For this review, take the finished solid that the model builds, in its own axes (mm). Face numbers are marked on the shaded views. A direction names the side the tool comes from. Round coordinates to 2 decimals unless told otherwise and drop trailing zeros. Order: outer loops, then holes, each group sorted by start corner. A loop starts at its lowest first (then second) coordinate and runs counter-clockwise, first axis right, second up.
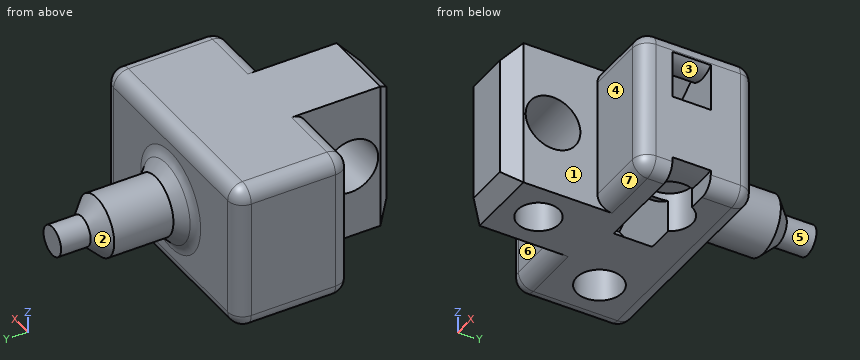
```python
from build123d import *

# Parameters (mm, degrees)
ESBO_O2_W                     = 100
ESBO_O2_H                     = 60
RESSALTO_EXTRUS_O1_DEPTH      = 50
RESSALTO_EXTRUS_O2_DEPTH      = 50
RESSALTO_EXTRUS_O2_DEPTH_BACK = 100
ESBO_O3_W                     = 100
ESBO_O3_H                     = 76.966331483
ESBO_O4_R                     = 20
RESSALTO_EXTRUS_O3_DEPTH      = 60
FILETE1_R                     = 10
CHANFRO1_SIZE                 = 10
ESBO_O6_R                     = 18.5
CORTE_EXTRUS_O1_DEPTH         = 243.47832014
ESBO_O7_R                     = 14.082818634
ESBO_O7_R_2                   = 15.375713497
CORTE_EXTRUS_O2_DEPTH         = 27
ESBO_O8_R                     = 10
RESSALTO_EXTRUS_O4_DEPTH      = 20
FILETE2_R                     = 10
CHANFRO2_SIZE                 = 10
ESBO_O10_W                    = 27.587633248
ESBO_O10_H                    = 25.966331483
ESBO_O10_W_2                  = 29.412366752
CORTE_REVOLU_O1_ANGLE         = 325


with BuildPart() as part:
    # Esboço2 → Ressalto-extrusão1 (new body)
    with BuildSketch(Plane(origin=(0, 0, 0), x_dir=(0, 0, -1), z_dir=(1, 0, 0))):
        with Locations((50, 30)):
            Rectangle(ESBO_O2_W, ESBO_O2_H)
    extrude(amount=RESSALTO_EXTRUS_O1_DEPTH)

    # Esboço3 → Ressalto-extrusão2 (add, two sides: drawn at the far end of the back side and taken through both)
    with BuildSketch(Plane.ZY.offset(-RESSALTO_EXTRUS_O2_DEPTH_BACK)):
        with Locations((-50, 98.483165742)):
            Rectangle(ESBO_O3_W, ESBO_O3_H)
    extrude(amount=RESSALTO_EXTRUS_O2_DEPTH + RESSALTO_EXTRUS_O2_DEPTH_BACK)

    # Esboço4 → Ressalto-extrusão3 (add)
    with BuildSketch(Plane(origin=(0, 136.966331483, 0), x_dir=(1, 0, 0), z_dir=(0, 1, 0))):
        with Locations(Location((25, 50, 0), (0, 0, 90))):
            Circle(ESBO_O4_R)
    extrude(amount=RESSALTO_EXTRUS_O3_DEPTH)

    # Filete1
    filete1_edges = [part.edges().sort_by_distance(p)[0] for p in [
        (-25, 60, -100),
        (75, 60, -100),
        (100, 60, -50),
        (-25, 60, 0),
        (75, 60, 0),
        (100, 98.483165742, 0),
        (25, 136.966331483, 0),
        (100, 136.966331483, -50),
        (25, 136.966331483, -100),
        (100, 98.483165742, -100),
        (-50, 60, -50),
        (-50, 98.483165742, 0),
        (-50, 136.966331483, -50),
        (-50, 98.483165742, -100),
    ]]
    fillet(filete1_edges, radius=FILETE1_R)

    # Chanfro1
    chanfro1_edges = [part.edges().sort_by_distance(p)[0] for p in [
        (25, 136.966331483, -30),
        (25, 196.966331483, -30),
    ]]
    chamfer(chanfro1_edges, length=CHANFRO1_SIZE)

    # Esboço6 → Corte-extrusão1 (cut, through all)
    with BuildSketch(Plane(origin=(50, 0, 0), x_dir=(0, 0, -1), z_dir=(1, 0, 0))):
        with Locations((50, 30)):
            Circle(ESBO_O6_R)
    extrude(amount=-CORTE_EXTRUS_O1_DEPTH, mode=Mode.SUBTRACT)

    # Esboço7 → Corte-extrusão2 (cut)
    with BuildSketch(Plane(origin=(0, 0, -100), x_dir=(-1, 0, 0), z_dir=(0, 0, -1))):
        with Locations((-25, 35)):
            Circle(ESBO_O7_R)
        with Locations((15, 99.947585823)):
            Circle(ESBO_O7_R_2)
        with Locations((-65, 99.947585823)):
            Circle(ESBO_O7_R_2)
    extrude(amount=-CORTE_EXTRUS_O2_DEPTH, mode=Mode.SUBTRACT)

    # Esboço8 → Ressalto-extrusão4 (add)
    with BuildSketch(Plane(origin=(0, 196.966331483, 0), x_dir=(1, 0, 0), z_dir=(0, 1, 0))):
        with Locations(Location((25, 50, 0), (0, 0, 270))):
            Circle(ESBO_O8_R)
    extrude(amount=RESSALTO_EXTRUS_O4_DEPTH)

    # Filete2
    filete2_edges = [part.edges().sort_by_distance(p)[0] for p in [
        (25, 136.966331483, -20),
    ]]
    fillet(filete2_edges, radius=FILETE2_R)

    # Chanfro2
    chanfro2_edges = [part.edges().sort_by_distance(p)[0] for p in [
        (50, 0, -50),
        (0, 0, -50),
        (25, 0, -100),
        (25, 0, 0),
    ]]
    chamfer(chanfro2_edges, length=CHANFRO2_SIZE)

    # Esboço10 → Corte-Revolução1 (revolve, cut)
    with BuildSketch(Plane.XY):
        with Locations((-11.206183376, 93.983165742)):
            Rectangle(ESBO_O10_W, ESBO_O10_H)
        with Locations((60.293816624, 93.983165742)):
            Rectangle(ESBO_O10_W_2, ESBO_O10_H)
    revolve(axis=Axis((90, 136.966331483, 0), (0, 1, 0)), revolution_arc=CORTE_REVOLU_O1_ANGLE, mode=Mode.SUBTRACT)


solid = part.part
```
Q1. Tool access review of the marked faces 4, 5, 6 and 7: name each direction out of +Z, -Z, +X, -X, +Y, -Y from which nothing blocks a thin tool from reaching the whole face with its end or side.
Q2. Wall thickness on line 1 (Y direction, x = 65, z = -79); line 2 (Y direction, x = 82.5, z = -24); line 3 (Y direction, x = 8.5, z = -63): over which ranges is each line inside the solid? List them lowest first.
Q3. Take a section at D-D, the plane y = 30. State the section outline as (x, z) points, plus the area to 3 significant figures.
Q4. Take a section at C-C, the plane z = -94. State the section outline as (x, y) points.
Q5. Mouldability with a two-part tool opening along Y and no side actions: class the marked faces 1, 2 and 3 as +Y half, -Y half, draft (parallel to the pull), parting line (faces both ways), or undercut.
Q6. Take a section at A-A, the plane x = 25. Count the separate pieces of the cut face and the enclosed holes in it, plus the area to 3 significant figures.
Q7. Take a section at B-B, the plane y = 90.5. State the section outline as (x, z) points, plus the area to 3 significant figures.
Q8. Clearance check with flat-ended pins moving along their axes: pin 1 (10.5 mm diameter, centred on x = 87.5, z = -96, fed in from -Y); pin 2 (14 mm diameter, centred on x = 22, y = 35.5, fed in from -Z); pin 3 (1 mm diameter, centred on y = 148, z = -39.5, fed in from +X). State where each tip first meets the part, or that it passes through.
Working result:
1. face 4: +Z, -Z, +X, -Y
1. face 5: +Y
1. face 6: +Z, -Z, -X, -Y
1. face 7: -Z, +X, -Y
2. line 1: y = 60 to 84.57, 115.32 to 136.97
2. line 2: y = 60 to 81, 106.97 to 136.97
2. line 3: y = 1.5 to 16.84, 43.16 to 81, 106.97 to 145.96
3. outline: (0, -100) - (11.83, -100) - (11.83, -73) - (38.17, -73) - (38.17, -100) - (50, -100) - (50, -68.5) - (0, -68.5) - close; (0, -31.5) - (50, -31.5) - (50, 0) - (0, 0) - close
3. area: 2,440 mm2
4. outline: (-49.17, 70) arc R9.17 ccw to (-40, 60.83) - (0, 60.83) - (0, 10) - (6, 4) - (44, 4) - (50, 10) - (50, 60.83) - (90, 60.83) arc R9.17 ccw to (99.17, 70) - (99.17, 81) - (23.75, 81) - (23.75, 106.97) - (51.32, 106.97) arc R15.38 cw to (78.68, 106.97) - (99.17, 106.97) - (99.17, 126.97) arc R9.17 ccw to (90, 136.13) - (-40, 136.13) arc R9.17 ccw to (-49.17, 126.97) - close; hole circle Ø30.75 at (-15, 99.95); hole circle Ø28.17 at (25, 35)
5. face 1: draft
5. face 2: +Y half
5. face 3: undercut
6. separate pieces: 1
6. enclosed holes: 2
6. area: 13,600 mm2
7. outline: (-50, -90) arc R10 ccw to (-40, -100) - (-27.13, -100) - (-27.13, -73) - (-2.87, -73) - (-2.87, -100) - (33.21, -100) arc R115 cw to (-4.2, -65.96) - (18.4, -50.14) arc R87.41 ccw to (52.87, -79.13) - (52.87, -73) - (77.13, -73) - (77.13, -86.46) arc R87.41 ccw to (100, -86.84) - (100, -43.27) arc R44.41 cw to (53.62, -25.47) - (77.71, -8.6) arc R15 ccw to (100, -11.18) - (100, -10) arc R10 ccw to (90, 0) - (-40, 0) arc R10 ccw to (-50, -10) - close
7. area: 10,700 mm2
8. pin 1: stops at y = 60.03
8. pin 2: stops at z = -73
8. pin 3: stops at x = 42.32
